Check sheet for the drawn part. Datum: minimum x, y, z corner. Units: mm. Round coordinates to 2 decimals unless told otherwise and drop trailing zeros. Order: outer loops, then holes, each group sorted by start corner. A loop starts at its lowest first (then second) coordinate and runs counter-clockwise, first axis right, second up. Notation, with made-up numbers: (87, 60.25) - (109, 60.25) arc R16 ccw to (109, 78.25) - close; hole circle Ø8 at (27.25, 12). An arc over 180 degrees is marked (long way). Write each question's results on one line, items separated by ' | '.
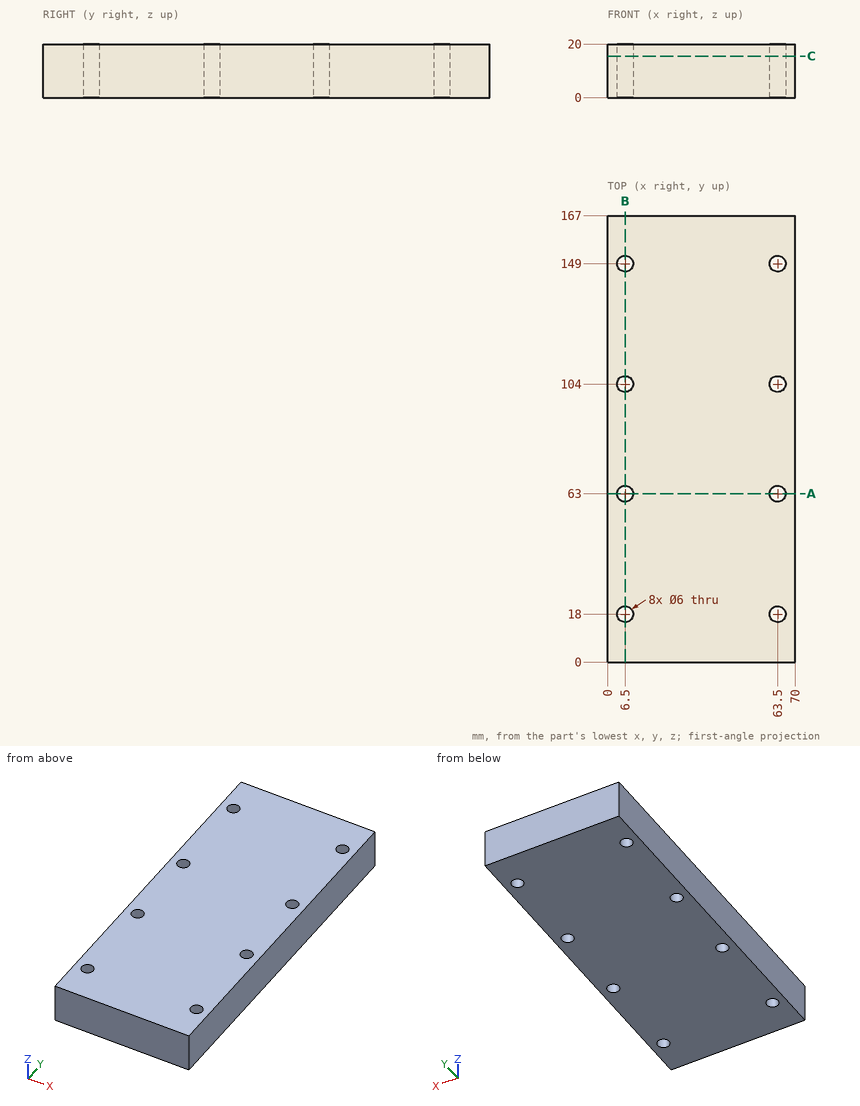
(1) Section check A-A (y = 63). Record the cut outline in (x, z), then the cut area to 3 significant figures.
Answers follow:
outline: (0, 0) - (3.5, 0) - (3.5, 20) - (0, 20) - close; (9.5, 0) - (60.5, 0) - (60.5, 20) - (9.5, 20) - close; (66.5, 0) - (70, 0) - (70, 20) - (66.5, 20) - close | area: 1,160 mm²
(2) Section check B-B (x = 6.5). Record the cut outline in (y, z), then the cut area to 3 significant figures.
Answers follow:
outline: (0, 0) - (15, 0) - (15, 20) - (0, 20) - close; (21, 0) - (60, 0) - (60, 20) - (21, 20) - close; (66, 0) - (101, 0) - (101, 20) - (66, 20) - close; (107, 0) - (146, 0) - (146, 20) - (107, 20) - close; (152, 0) - (167, 0) - (167, 20) - (152, 20) - close | area: 2,860 mm²
(3) Section check C-C (z = 15.5). Give the number of separate pieces and of enclosed holes in the cut face, then the cut area to 3 significant figures.
Answers follow:
separate pieces: 1 | enclosed holes: 8 | area: 11,500 mm²
(4) Material ranges on line 1 (Y direction, x = 63.5, z = 7); line 2 (X direction, y = 149, z = 15.75); line 3 (Y direction, x = 5, z = 9.25), recorded low to high.
Answers follow:
line 1: 0 to 15, 21 to 60, 66 to 101, 107 to 146, 152 to 167 | line 2: 0 to 3.5, 9.5 to 60.5, 66.5 to 70 | line 3: 0 to 15.4, 20.6 to 60.4, 65.6 to 101.4, 106.6 to 146.4, 151.6 to 167
